CAD build for the part. Positions are in the model's coordinates, mm. A direction names the side the tool comes from. Round coordinates to 2 decimals unless told otherwise and drop trailing zeros. Order: outer loops, then holes, each group sorted by start corner. A loop starts at its lowest first (then second) coordinate and runs counter-clockwise, first axis right, second up. Notation, with made-up numbers: M -19.5,89 L 37.5,89 A26 ccw 37.5,106 Z; hole C -36.5,11 d10. An arc over 180 degrees is marked long. Answer as a JSON object with one key per item and string values.
```python
from build123d import *

# Parameters (mm, degrees)
SKETCH1_R           = 25
BOSS_EXTRUDE1_DEPTH = 5
SKETCH2_R           = 30
BOSS_EXTRUDE2_DEPTH = 25
SKETCH3_W           = 20
SKETCH3_H           = 40
BOSS_EXTRUDE3_DEPTH = 50
CHAMFER1_SIZE       = 10
SKETCH5_R           = 12.5
CUT_EXTRUDE1_DEPTH  = 91.138781887


with BuildPart() as part:
    # Sketch1 → Boss-Extrude1 (new body)
    with BuildSketch(Plane.XY):
        Circle(SKETCH1_R)
    extrude(amount=BOSS_EXTRUDE1_DEPTH)

    # Sketch2 → Boss-Extrude2 (add)
    with BuildSketch(Plane(origin=(0, 0, 0), x_dir=(-1, 0, 0), z_dir=(0, 0, -1))):
        Circle(SKETCH2_R)
    extrude(amount=BOSS_EXTRUDE2_DEPTH)

    # Sketch3 → Boss-Extrude3 (add)
    with BuildSketch(Plane(origin=(0, 0, -25), x_dir=(-1, 0, 0), z_dir=(0, 0, -1))):
        Rectangle(SKETCH3_W, SKETCH3_H)
    extrude(amount=BOSS_EXTRUDE3_DEPTH)

    # Chamfer1
    chamfer1_edges = [part.edges().sort_by_distance(p)[0] for p in [
        (0, 20, -75),
        (0, -20, -75),
    ]]
    chamfer(chamfer1_edges, length=CHAMFER1_SIZE)

    # Sketch5 → Cut-Extrude1 (cut, through all)
    with BuildSketch(Plane.ZY.offset(10)):
        with Locations((-55, 0)):
            Circle(SKETCH5_R)
    extrude(amount=-CUT_EXTRUDE1_DEPTH, mode=Mode.SUBTRACT)


solid = part.part
```
Item 1: Saw through at B-B on z = -55. List the corners of the cut face in (x, y), and give its area (3 significant figures).
Worked answers:
{"outline": "M -10,-20 L 10,-20 L 10,-12.5 L -10,-12.5 Z; M -10,12.5 L 10,12.5 L 10,20 L -10,20 Z", "area": "300 mm2"}
Item 2: Saw through at D-D on x = 24. List the corners of the cut face in (y, z).
Worked answers:
{"outline": "M -18,-25 L 18,-25 L 18,0 L 7,0 L 7,5 L -7,5 L -7,0 L -18,0 Z"}
Item 3: Saw through at A-A on y = 0. List the corners of the cut face in (x, z).
Worked answers:
{"outline": "M -30,-25 L -10,-25 L -10,-42.5 L 10,-42.5 L 10,-25 L 30,-25 L 30,0 L 25,0 L 25,5 L -25,5 L -25,0 L -30,0 Z; M -10,-75 L 10,-75 L 10,-67.5 L -10,-67.5 Z"}
Item 4: Wall check: line 1 along Y through (x, z) = (-4.25, -55); line 2 along Y through (x, z) = (1, -28.5); line 3 along X through (y, z) = (-11.5, -34.5). Give the ranges that are in metal, low to high. Write a range as [from, to].
Worked answers:
{"line 1": "y = [-20, -12.5], [12.5, 20]", "line 2": "y = [-20, 20]", "line 3": "x = [-10, 10]"}
Item 5: Saw through at C-C on x = 0. List the corners of the cut face in (y, z).
Worked answers:
{"outline": "M -30,-25 L -20,-25 L -20,-65 L -10,-75 L 10,-75 L 20,-65 L 20,-25 L 30,-25 L 30,0 L 25,0 L 25,5 L -25,5 L -25,0 L -30,0 Z; hole C 0,-55 d25"}
Item 6: Drop flat-ended pins along their axis: pin 1 Ø6 at (y, z) = (-1, -22) entering from +X; pin 2 Ø1 at (x, y) = (-15.5, 21) entering from -Z; pin 3 Ø6 at (x, z) = (1.5, -47.5) entering from +Y; pin 4 Ø8 at (y, z) = (-17.5, -66.5) entering from -X. Give the stop position or say it passes through.
Worked answers:
{"pin 1": "stops at x = 30", "pin 2": "stops at z = -25", "pin 3": "stops at y = 20", "pin 4": "stops at x = -10"}
Item 7: Two-plate mould, pull along Y, no slides. Class faces 1 (the cylindrical face through (-0.14, 0.55, -67.488)), 2 (the flat face through (0, -20, -45)), 3 (the flat face through (0, 15, -70)): released by +Y, released by -Y, zero draft, split by the parting line, or undercut.
Worked answers:
{"face 1": "undercut", "face 2": "released by -Y", "face 3": "released by +Y"}
Item 8: 3-axis set-ups, long thin cutter, end or side, ignore diameter. For faces 4 (the flat face through (10, 0, -39)), 5 (the flat face through (0, 20, -45)), 6 (the flat face through (7, 25, 0)): which of +Z, -Z, +X, -X, +Y, -Y reach the whole face in a straight line?
Worked answers:
{"face 4": "-Z, +X, +Y, -Y", "face 5": "-Z, +X, -X, +Y", "face 6": "+Z"}
